Could you check a few things on this drawing? It's one solid part, dimensions in mm from its lowest x, y, z. Round coordinates to 2 decimals unless told otherwise and drop trailing zeros. Write each loop counter-clockwise with the first axis right and the second up, starting at its lowest first coordinate (ties: lowest second). Pieces come first, ordered by that corner, then holes. Notation, with made-up numbers: (84, 9.5) - (101, 9.5) arc R26 ccw to (101, 43.5) - close; hole circle Ø7 at (67.5, -7). An arc over 180 degrees is marked (long way). Write item = value, one per line. Start each with the question number.
Item 1: If we section it at B-B (x = 40): Please give me the cut outline in (y, z) (1 decimal).
Item 2: If we section it at A-A (y = 25.4): Please give me the cut outline in (x, z) (1 decimal).
Item 3: If I drill on line 1 along Y through (x, z) = (25.4, 70) (1 decimal); line 2 along X through (y, z) = (25, 90.5); line 3 along X through (y, z) = (33, 22.5) (1 decimal), over which ranges is the centre line in solid material (lowest first)? Write a range as [from, to].
Item 4: For P1, Ø2, axis at y = 28.5, z = 50, coming from the -X side; P2, Ø6, axis at x = 13, y = 31, coming from the +Z side; P3, Ø3, axis at x = 18, z = 51.5, coming from the +Y side (1 decimal); P4, Ø1.5, axis at x = 26.5, z = 39.5, coming from the +Y side, each with a flat end and sliding along its axis, tell me the tip position at first contact or that it passes through.
Item 5: Thinking about a two-plate mould opening in X: for the marked faces 1, 2 and 3, which applies, pulls with the +X half, pulls with the -X half, needs draft (parallel to the pull), parting line crosses it, or undercut?
Item 6: If we section it at D-D (x = 8): Please give me the cut outline in (y, z) (1 decimal), and give its area (3 significant figures).
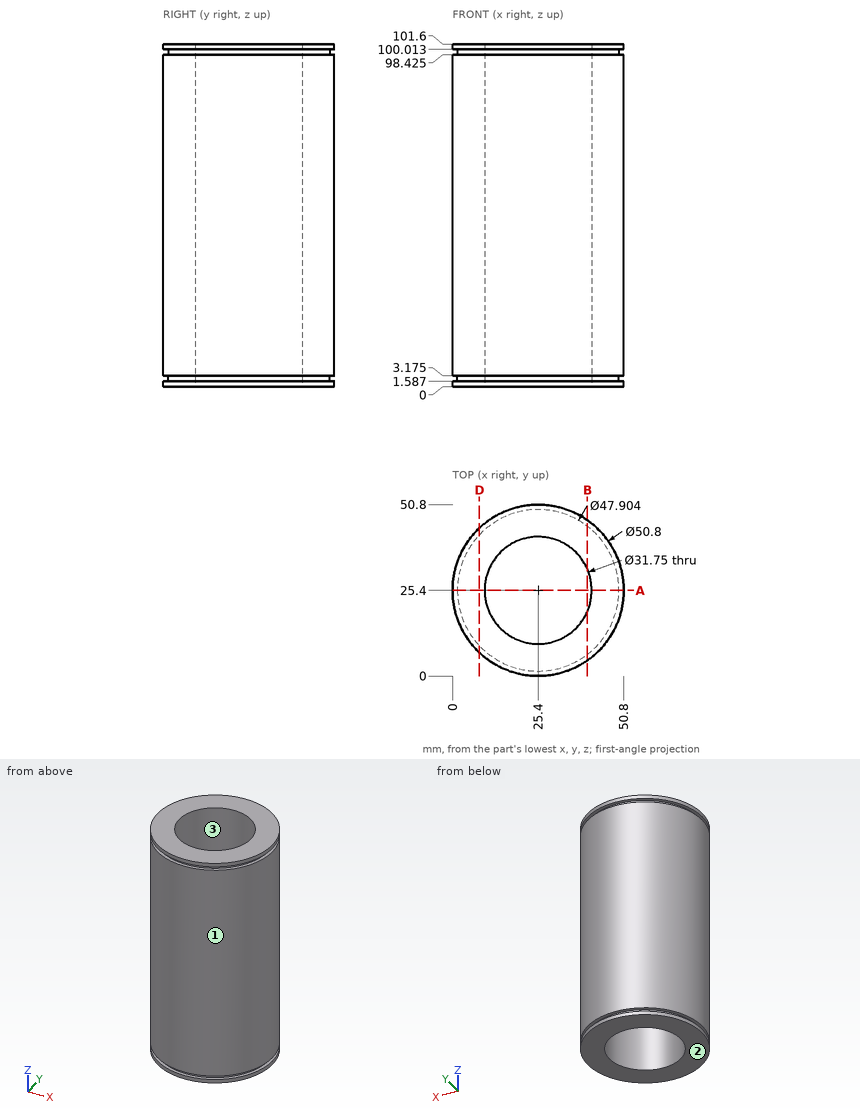
Reply:
q1.outline = (4.6, 0) - (19.2, 0) - (19.2, 101.6) - (4.6, 101.6) - (4.6, 100) - (6.4, 100) - (6.4, 98.4) - (4.6, 98.4) - (4.6, 3.2) - (6.4, 3.2) - (6.4, 1.6) - (4.6, 1.6) - close; (31.6, 0) - (46.2, 0) - (46.2, 1.6) - (44.4, 1.6) - (44.4, 3.2) - (46.2, 3.2) - (46.2, 98.4) - (44.4, 98.4) - (44.4, 100) - (46.2, 100) - (46.2, 101.6) - (31.6, 101.6) - close
q2.outline = (0, 0) - (9.5, 0) - (9.5, 101.6) - (0, 101.6) - (0, 100) - (1.4, 100) - (1.4, 98.4) - (0, 98.4) - (0, 3.2) - (1.4, 3.2) - (1.4, 1.6) - (0, 1.6) - close; (41.3, 0) - (50.8, 0) - (50.8, 1.6) - (49.4, 1.6) - (49.4, 3.2) - (50.8, 3.2) - (50.8, 98.4) - (49.4, 98.4) - (49.4, 100) - (50.8, 100) - (50.8, 101.6) - (41.3, 101.6) - close
q3.line_1 = [0, 9.5], [41.3, 50.8]
q3.line_2 = [0, 9.53], [41.27, 50.8]
q3.line_3 = [1.2, 11.5], [39.3, 49.6]
q4.P1 = 0.09
q4.P2 = 101.6
q4.P3 = 50.1
q4.P4 = 50.8
q5.face_1 = parting line crosses it
q5.face_2 = needs draft
q5.face_3 = undercut
q6.outline = (6.9, 0) - (43.9, 0) - (43.9, 1.6) - (41.9, 1.6) - (41.9, 3.2) - (43.9, 3.2) - (43.9, 98.4) - (41.9, 98.4) - (41.9, 100) - (43.9, 100) - (43.9, 101.6) - (6.9, 101.6) - (6.9, 100) - (8.9, 100) - (8.9, 98.4) - (6.9, 98.4) - (6.9, 3.2) - (8.9, 3.2) - (8.9, 1.6) - (6.9, 1.6) - close
q6.area = 3,750 mm2
